from build123d import *

# Parameters (mm, degrees)
BOSS_EXTRUDE1_DEPTH = 1
SKETCH2_R           = 2
BOSS_EXTRUDE2_DEPTH = 4


with BuildPart() as part:
    # Sketch1 → Boss-Extrude1 (new body)
    with BuildSketch(Plane(origin=(0, 0, 0), x_dir=(1, 0, 0), z_dir=(0, 1, 0))):
        with BuildLine():
            Line((-3.5, 2), (-6.5, 2))
            ThreePointArc((-6.5, 2), (-8.5, 0), (-6.5, -2))
            Line((-6.5, -2), (-3, -2))
            Line((-3, -2), (-2, -14))
            ThreePointArc((-2, -14), (0, -16), (2, -14))
            Line((2, -14), (3, -2))
            Line((3, -2), (6.5, -2))
            ThreePointArc((6.5, -2), (8.5, 0), (6.5, 2))
            Line((6.5, 2), (3.5, 2))
            Line((3.5, 2), (2, 17))
            ThreePointArc((2, 17), (0, 19), (-2, 17))
            Line((-2, 17), (-3.5, 2))
        make_face()
    extrude(amount=BOSS_EXTRUDE1_DEPTH)

    # Sketch2 → Boss-Extrude2 (add)
    with BuildSketch(Plane(origin=(0, 1, 0), x_dir=(1, 0, 0), z_dir=(0, 1, 0))):
        Circle(SKETCH2_R)
    extrude(amount=BOSS_EXTRUDE2_DEPTH)


solid = part.part
Build history of the part. All positions in model axes, mm. A direction names the side the tool comes from. Give positions to 0.01 mm unless a question says otherwise; leave off trailing zeros. Order: outer loops, then holes, each group sorted by start corner. A loop starts at its lowest first (then second) coordinate and runs counter-clockwise, first axis right, second up. Notation, with made-up numbers: M 19.5,-40 L 39.5,-40 A16 cw 39.5,-20 Z; hole C 46,-18 d5. An arc over 180 degrees is marked long. Put each result on its own line as item: value.
Item 1: Pull direction X, two halves, no side cores. Call faces 4 (the face through (2.493, 0.493, 8.084)), 5 (the face through (-2.507, 0.493, 7.916)), 6 (the face through (0, 0, -2)): +X half, -X half, draft (parallel to the pull), parting line (faces both ways), or undercut.
Results are:
face 4: +X half
face 5: -X half
face 6: draft
Item 2: Cut at A-A on x = 0. Write the cut outline in (y, z).
Results are:
outline: M 0,-19 L 1,-19 L 1,-2 L 5,-2 L 5,2 L 1,2 L 1,16 L 0,16 Z
Item 3: Wall check: probe 1 along Y at (x, z) = (-6.5, 0); probe 2 along Z at (x, y) = (-6.5, 0.3); probe 3 along X at (y, z) = (0.8, 9). Give the ranges that are in metal, low to high.
Results are:
probe 1: 0 to 1
probe 2: -2 to 2
probe 3: -2.42 to 2.42
Item 4: Which spindle directions (+Z, -Z, +X, -X, +Y, -Y) get a long thin tool onto all of the face, cutting with end or side? Do faces 1 (the face through (0, 3, 2)), 2 (the face through (-4.8, 0.5, 2)), 3 (the face through (5, 0.5, -2)). Say none if no direction does.
Results are:
face 1: +Y
face 2: +Z, -X, +Y, -Y
face 3: -Z, +X, +Y, -Y
Item 5: Cut at D-D on z = -10. Write the cut outline in (x, y), then the cut area to 3 significant figures.
Results are:
outline: M -2.7,0 L 2.7,0 L 2.7,1 L -2.7,1 Z
area: 5.40 mm2
Item 6: Drop flat-ended pins along their axis: pin 1 Ø2 at (y, z) = (2.5, 2) entering from +X; pin 2 Ø0.5 at (x, y) = (-4.5, 0.5) entering from +Z; pin 3 Ø8 at (x, z) = (4, -11) entering from +Y. Give the stop position or say it passes through.
Results are:
pin 1: x = 1.73
pin 2: z = 2
pin 3: y = 1
Item 7: Cut at C-C on y = 2. Write the cut outline in (x, z).
Results are:
outline: C 0,0 d4
Item 8: Cut at B-B on z = 11. Write the cut outline in (x, y).
Results are:
outline: M -2.25,0 L 2.25,0 L 2.25,1 L -2.25,1 Z
